For this review, use the dimensioned drawing (mm, ordinates from the lowest corner) and the shaded views. A direction names the side the tool comes from. Coordinates: 2 decimals unless noted, no trailing zeros. Order: outer loops, then holes, each group sorted by start corner. A loop starts at its lowest first (then second) coordinate and runs counter-clockwise, first axis right, second up. Notation, with made-up numbers: (72, -38) -> (117, -38) arc R33 ccw to (117, -4) -> close; hole circle Ø10 at (26.25, 74.25). An arc over 180 degrees is marked (long way). Use one line per item in the form item = value. Start each with the question number.
(1) Take a section at B-B (y = 28). State the section outline as (x, z) points, then the cut area to 3 significant figures.
(2) For the marked faces 1, 2 and 3, list the 3-axis set-ups (+Z, -Z, +X, -X, +Y, -Y) from which the entire face can be reached by the end or side of a thin tool; tool diameter is ignored.
(3) Take a section at A-A (z = 37). State the section outline as (x, y) points, then the cut area to 3 significant figures.
(4) Wall thickness on line 1 along X through (y, z) = (7.5, 29); line 2 along Z through (x, y) = (5, 9); line 3 along Z through (x, y) = (32.5, 46.5): over which ranges is each line inside the solid? List them lowest first.
(5) Take a section at D-D (z = 4.5). State the section outline as (x, y) points.
(6) Take a section at C-C (x = 3.5). State the section outline as (y, z) points, then the cut area to 3 significant figures.
(7) Mouldability with a two-part tool opening along X and no side actions: class the marked faces 4, 5 and 6 as +X half, -X half, draft (parallel to the pull), parting line (faces both ways), or undercut.
(8) Insertion check: pin 1 Ø4 at (x, z) = (26, 9.5) entering from +Y; pin 2 Ø2 at (y, z) = (22, 16) entering from +X; pin 3 Ø5 at (x, y) = (9.5, 37) entering from -Z; pin 4 Ø12 at (y, z) = (24, 21.5) entering from -X. Each pin has a flat end and moves straight along its axis. Give the tip position at first contact, or say it passes through.
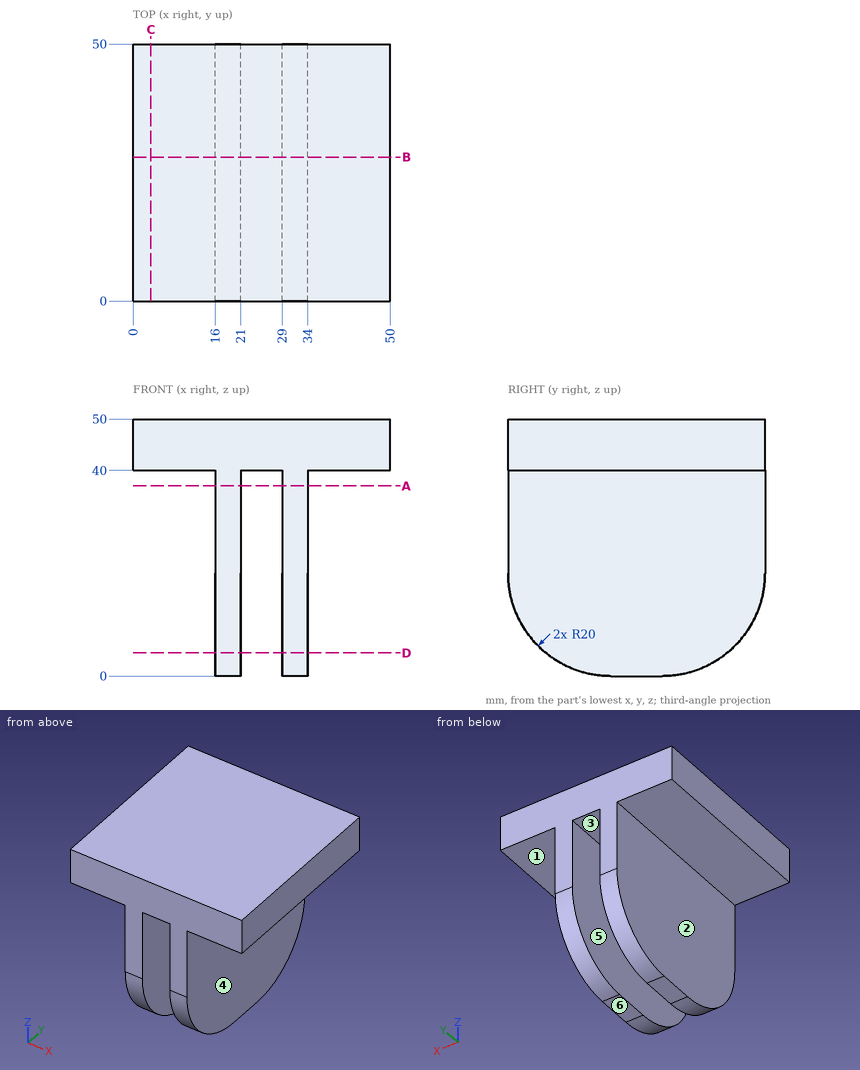
Findings:
q1.outline = (0, 40) -> (16, 40) -> (16, 0) -> (21, 0) -> (21, 40) -> (29, 40) -> (29, 0) -> (34, 0) -> (34, 40) -> (50, 40) -> (50, 50) -> (0, 50) -> close
q1.area = 900 mm²
q2.face_1 = -Z, +X, +Y, -Y
q2.face_2 = -Z, -X, +Y, -Y
q2.face_3 = -Z, +Y, -Y
q3.outline = (16, 0) -> (21, 0) -> (21, 50) -> (16, 50) -> close; (29, 0) -> (34, 0) -> (34, 50) -> (29, 50) -> close
q3.area = 500 mm²
q4.line_1 = 16 to 21, 29 to 34
q4.line_2 = 40 to 50
q4.line_3 = 8.7 to 50
q5.outline = (16, 7.36) -> (21, 7.36) -> (21, 42.64) -> (16, 42.64) -> close; (29, 7.36) -> (34, 7.36) -> (34, 42.64) -> (29, 42.64) -> close
q6.outline = (0, 40) -> (50, 40) -> (50, 50) -> (0, 50) -> close
q6.area = 500 mm²
q7.face_4 = +X half
q7.face_5 = undercut
q7.face_6 = draft
q8.pin_1 = through
q8.pin_2 = 34
q8.pin_3 = 40
q8.pin_4 = 16
